```python
from build123d import *

# Parameters (mm, degrees)
F0_W     = 192.8
F0_H     = 71.8
F0_W_2   = 188
F0_H_2   = 67
F1_DEPTH = 35
F2_R     = 3
F3_DEPTH = 192.801
F4_R     = 3.9
F5_DEPTH = 25
F6_R     = 3
F7_DEPTH = 25


with BuildPart() as f1:
    # F0 (on Top) → F1 (new body)
    with BuildSketch(Plane.XY):
        Rectangle(F0_W, F0_H)
        Rectangle(F0_W_2, F0_H_2, mode=Mode.SUBTRACT)
    extrude(amount=F1_DEPTH)

    # F2 (on face) → F3 (cut, through all)
    with BuildSketch(Plane(origin=(-96.4, 0, 0), x_dir=(0, -1, 0), z_dir=(-1, 0, 0))):
        with Locations((-17.95, 17.5)):
            Circle(F2_R)
        with Locations((17.95, 17.5)):
            Circle(F2_R)
    extrude(amount=-F3_DEPTH, mode=Mode.SUBTRACT)

    # F4 (on face) → F5 (cut)
    with BuildSketch(Plane.XZ.offset(35.9)):
        with Locations((0, 17.5)):
            Circle(F4_R)
        with Locations((33, 17.5)):
            Circle(F4_R)
        with Locations((66, 17.5)):
            Circle(F4_R)
        with Locations((-33, 17.5)):
            Circle(F4_R)
        with Locations((-66, 17.5)):
            Circle(F4_R)
    extrude(amount=-F5_DEPTH, mode=Mode.SUBTRACT)

    # F6 (on face) → F7 (cut)
    with BuildSketch(Plane(origin=(0, 35.9, 0), x_dir=(-1, 0, 0), z_dir=(0, 1, 0))):
        with Locations((0, 17.5)):
            Circle(F6_R)
        with Locations((33, 17.5)):
            Circle(F6_R)
        with Locations((66, 17.5)):
            Circle(F6_R)
        with Locations((-33, 17.5)):
            Circle(F6_R)
        with Locations((-66, 17.5)):
            Circle(F6_R)
    extrude(amount=-F7_DEPTH, mode=Mode.SUBTRACT)


solid = f1.part
```
Check sheet for the modelled part. Datum: model origin and axes. Units: mm. A direction names the side the tool comes from. Give positions to 0.01 mm unless a question says otherwise; leave off trailing zeros. Loops run counter-clockwise (first coordinate to the right, second up) from the corner with the lowest first, then second, coordinate; pieces in that order, holes last. Notation, with made-up numbers: (-31.75, 21) - (6.25, 21) arc R21 cw to (6.25, 26) - close; hole circle Ø6 at (-12, 27). An arc over 180 degrees is marked (long way). One line per question, with ' | ' between items. Start each with the question number.
1. Cross-section at D-D, the plane z = 28.5. Enter the section's corners in (x, y).
2. Cross-section at B-B, the plane y = 17.95. Enter the section's corners in (x, z).
3. Cross-section at C-C, the plane x = 19.5. Enter the section's corners in (y, z).
4. Set-up check for faces 4 (the flat face through (-1, -33.5, 13)), 5 (the cylindrical face through (-36.896, -34.717, 17.671)), 6 (the cylindrical face through (-30.6, 34.7, 15.7)): record each of +Z, -Z, +X, -X, +Y, -Y from which the full face is reachable in a straight line by a thin tool's end or side.
5. Cross-section at A-A, the plane y = -12. Enter the section's corners in (x, z).
6. Material ranges on line 1 along X through (y, z) = (-35, 17); line 2 along Z through (x, y) = (0, 34); line 3 along X through (y, z) = (7, 27), recorded low to high. Write a range as [from, to].
7. Draft check along X on faces 1 (the flat face through (0, 35, 35)), 2 (the cylindrical face through (29.104, -34.717, 17.671)), 3 (the flat face through (-96.4, -1, 17)). Enter one of: released by +X, released by -X, zero draft, split by the parting line, or undercut.
8. Gauge pin test, flat ends, axial feed: pin 1 Ø7 at (x, z) = (-33, 17.5) entering from +Y; pin 2 Ø7 at (x, z) = (0, 17.5) entering from -Y. Record the tip position at first contact, or that the pin passes through.
Check result:
1) outline: (-96.4, -35.9) - (96.4, -35.9) - (96.4, 35.9) - (-96.4, 35.9) - close; hole (-94, -33.5) - (94, -33.5) - (94, 33.5) - (-94, 33.5) - close
2) outline: (-96.4, 0) - (-94, 0) - (-94, 14.5) - (-96.4, 14.5) - close; (-96.4, 20.5) - (-94, 20.5) - (-94, 35) - (-96.4, 35) - close; (94, 0) - (96.4, 0) - (96.4, 14.5) - (94, 14.5) - close; (94, 20.5) - (96.4, 20.5) - (96.4, 35) - (94, 35) - close
3) outline: (-35.9, 0) - (-33.5, 0) - (-33.5, 35) - (-35.9, 35) - close; (33.5, 0) - (35.9, 0) - (35.9, 35) - (33.5, 35) - close
4) face 4: +Z, -Z | face 5: -Y | face 6: +Y, -Y
5) outline: (-96.4, 0) - (-94, 0) - (-94, 35) - (-96.4, 35) - close; (94, 0) - (96.4, 0) - (96.4, 35) - (94, 35) - close
6) line 1: x = [-96.4, -69.87], [-62.13, -36.87], [-29.13, -3.87], [3.87, 29.13], [36.87, 62.13], [69.87, 96.4] | line 2: z = [0, 14.5], [20.5, 35] | line 3: x = [-96.4, -94], [94, 96.4]
7) face 1: zero draft | face 2: undercut | face 3: released by -X
8) pin 1: stops at y = 35.9 | pin 2: stops at y = 33.5
